from build123d import *

# Parameters (mm, degrees)
RECPAT_COUNT = 2
RECPAT_ANGLE = 90


with BuildPart() as part:
    # BodySke → Base-Revolve (revolve)
    with BuildSketch(Plane.XY, mode=Mode.PRIVATE) as base_revolve_sk:
        Polygon((0, 0), (0, 4.2), (0.15, 4.2), (2.7, 1.65), (10, 1.65), (10, 0), align=None)
    revolve(base_revolve_sk.sketch.rotate(Axis((-6.35, 0, 0), (1, 0, 0)), 90), axis=Axis((-6.35, 0, 0), (1, 0, 0)))

    # Sketch3 → Recess section 0
    with BuildSketch(Plane.ZY):
        with BuildLine():
            Line((-0.515, 2.2), (0.515, 2.2))
            Line((0.515, 2.2), (0.515, -2.2))
            Line((0.515, -2.2), (-0.515, -2.2))
            Line((-0.515, -2.2), (-0.515, 2.2))
        make_face()
    # Sketch4 → Recess section 1
    with BuildSketch(Plane.ZY.offset(-2.51)):
        with BuildLine():
            Line((-0.515, 0.948560373), (0.515, 0.948560373))
            Line((0.515, 0.948560373), (0.515, -0.948560373))
            Line((0.515, -0.948560373), (-0.515, -0.948560373))
            Line((-0.515, -0.948560373), (-0.515, 0.948560373))
        make_face()
    recess = loft(mode=Mode.SUBTRACT)

    # RecPat: Recess ×2 about axis
    recpat_axis = Axis((0, 0, 0), (1, 0, 0))
    for i in range(1, RECPAT_COUNT):
        add(recess.rotate(recpat_axis, i * RECPAT_ANGLE / (RECPAT_COUNT - 1)), mode=Mode.SUBTRACT)

    # RecCorSke → RecessCore (revolve, cut)
    with BuildSketch(Plane.XY, mode=Mode.PRIVATE) as recesscore_sk:
        Polygon((0, 0), (0, 1.026516298), (2.51, 0.851), (2.786506661, 0), align=None)
    revolve(recesscore_sk.sketch.rotate(Axis((-3.175, 0, 0), (1, 0, 0)), 90), axis=Axis((-3.175, 0, 0), (1, 0, 0)), mode=Mode.SUBTRACT)


solid = part.part
The listing builds one solid part. Answer for the finished solid, in the listing's coordinates (mm). A direction names the side the tool comes from. Coordinates: 2 decimals unless noted, no trailing zeros. Write each loop counter-clockwise with the first axis right and the second up, starting at its lowest first coordinate (ties: lowest second). Pieces come first, ordered by that corner, then holes. Notation, with made-up numbers: M 79.25,-23 L 128.25,-23 A23 ccw 128.25,12 Z; hole C -19.5,-14 d3. An arc over 180 degrees is marked long. Put each result on its own line as item: value. Start each with the question number.
1. For a pull along Y with two mould halves and no side action, classify faces 4 (the flat face through (0, 1, -1)), 5 (the conical face through (2.77, 0.04, 0.02)), 6 (the conical face through (2.58, -0.53, 1.69)) as pulls with the +Y half, pulls with the -Y half, needs draft (parallel to the pull), parting line crosses it, or undercut.
2. Which of the six approach directions +Z, -Z, +X, -X, +Y, -Y give full straight-line access (tool end or side, diameter ignored) to faces 1 (the cylindrical face through (6.401, -1.115, -1.216)), 2 (the flat face through (10, 0, 0)), 3 (the flat face through (1.273, 0.007, 1.566))?
3. Consider line 1 (Z direction, x = 2, y = 1) (3 decimals); line 2 (Y direction, x = 4, z = 0.5); line 3 (X direction, y = -0.25, z = -1.25). Determine where each line is inside the solid, lowest interval first. Write a range as from..to.
4. A cutting plane is placed at A-A on x = 4.25. Write down the section's boundary in (y, z).
5. Flat-ended cylindrical pins translate along their axes: P1, Ø1.5, axis at x = 2, z = 2, coming from the +Y side; P2, Ø5, axis at x = 5, y = -1, coming from the +Z side; P3, Ø1, axis at x = 8, y = 2.5, coming from the +Z side; P4, Ø1, axis at y = 3, z = 1.5, coming from the +X side. Find the tip coordinate at first contact, or state that the pin passes through.
Resolved:
1. face 4: needs draft
1. face 5: undercut
1. face 6: parting line crosses it
2. face 1: +X
2. face 2: +Z, -Z, +X, +Y, -Y
2. face 3: -X
3. line 1: z = -2.127..-0.515, 0.515..2.127
3. line 2: y = -1.57..1.57
3. line 3: x = 1.91..10
4. outline: C 0,0 d3.3
5. P1: stops at y = 2.52
5. P2: stops at z = 1.73
5. P3: passes through
5. P4: stops at x = 1.5
